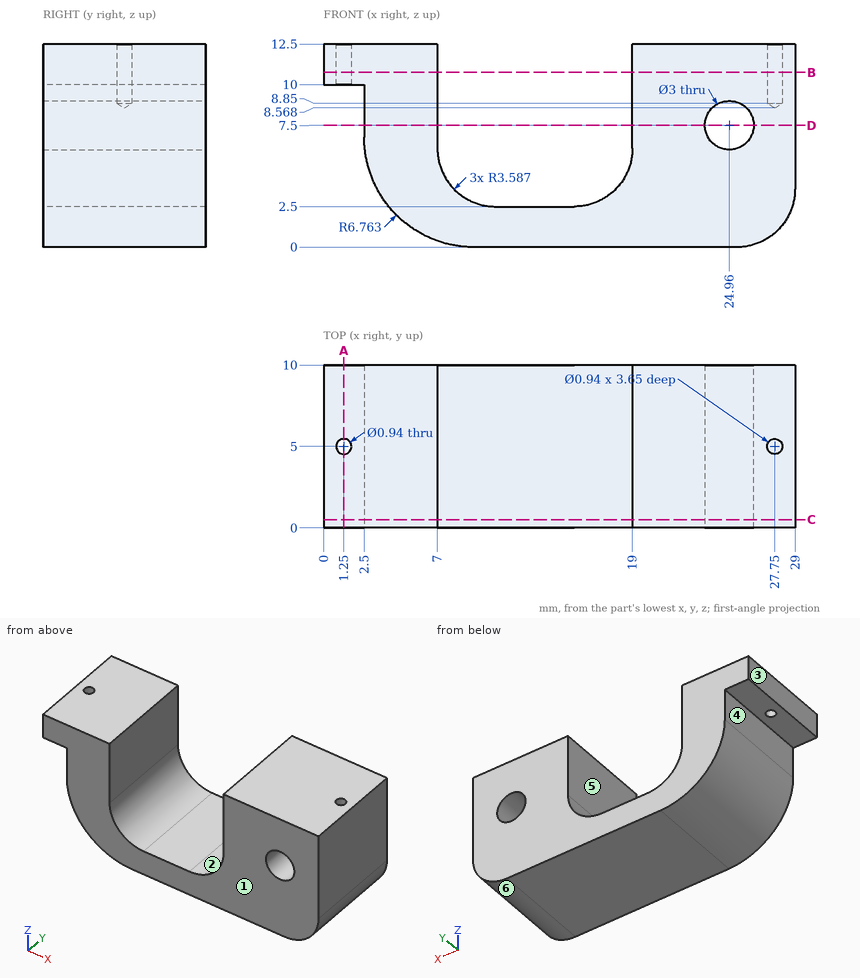
Study the drawing (mm; zero at the part's minimum x, y, z) and answer. A direction names the side the tool comes from. Round coordinates to 2 decimals unless told otherwise and drop trailing zeros. Write each loop counter-clockwise with the first axis right and the second up, starting at its lowest first coordinate (ties: lowest second). Pieces come first, ordered by that corner, then holes. Notation, with made-up numbers: (43, 73.5) - (48, 73.5) arc R19 ccw to (48, 94.5) - close; hole circle Ø4 at (-10.75, 26.25). An arc over 180 degrees is marked (long way). Use a Markdown table: item, result. Add a question column.
1. The part is cut by section C-C (y = 0.5). Write down the section's boundary in (x, z) (1 decimal), and give its area (3 significant figures).
2. The part is cut by section B-B (z = 10.75). Write down the section's boundary in (x, y).
3. The part is cut by section D-D (z = 7.5). Write down the section's boundary in (x, y), and give its area (3 significant figures).
4. The part is cut by section A-A (x = 1.25). Write down the section's boundary in (y, z).
5. Flat-ended cylindrical pins translate along their axes: P1, Ø5.5, axis at x = 13, y = 3, coming from the +Z side; P2, Ø2, axis at x = 8.5, y = 8.5, coming from the +Z side; P3, Ø6, axis at x = 3.5, y = 7.5, coming from the -Z side. Find the tip coordinate at first contact, or state that the pin passes through.
6. A tool of negligible diameter and unlimited length cuts with its end or side. For the marked faces 4, 5 and 6, from which of +Z, -Z, +X, -X, +Y, -Y can it reach the whole face along a straight path? Write none if from no direction.
7. Consider line 1 (X direction, y = 5, z = 10.5); line 2 (Z direction, x = 24.96, y = 3.25); line 3 (Y direction, x = 1.25, z = 11.3). Determine where each line is inside the solid, lowest interval first.
8. For a pull along X with two mould halves and no side action, classify the marked faces 1, 2 and 3 as +X half, -X half, draft (parallel to the pull), parting line (faces both ways), or undercut.
Reported:
| question | item | result |
|---|---|---|
| 1 | outline | (0, 10) - (2.5, 10) - (2.5, 6.8) arc R6.8 ccw to (9.3, 0) - (25.4, 0) arc R3.6 ccw to (29, 3.6) - (29, 12.5) - (19, 12.5) - (19, 6.1) arc R3.6 cw to (15.4, 2.5) - (10.6, 2.5) arc R3.6 cw to (7, 6.1) - (7, 12.5) - (0, 12.5) - close; hole circle Ø3 at (25, 7.5) |
| 1 | area | 203 mm^2 |
| 2 | outline | (0, 0) - (7, 0) - (7, 10) - (0, 10) - close; (19, 0) - (29, 0) - (29, 10) - (19, 10) - close; hole circle Ø0.94 at (1.25, 5); hole circle Ø0.94 at (27.75, 5) |
| 3 | outline | (2.5, 0) - (7, 0) - (7, 10) - (2.5, 10) - close; (19, 0) - (23.46, 0) - (23.46, 10) - (19, 10) - close; (26.46, 0) - (29, 0) - (29, 10) - (26.46, 10) - close |
| 3 | area | 115 mm^2 |
| 4 | outline | (0, 10) - (4.53, 10) - (4.53, 12.5) - (0, 12.5) - close; (5.47, 10) - (10, 10) - (10, 12.5) - (5.47, 12.5) - close |
| 5 | P1 | z = 2.52 |
| 5 | P2 | z = 4.26 |
| 5 | P3 | z = 0.59 |
| 6 | face 4 | -Z, -X, +Y, -Y |
| 6 | face 5 | +Z, +Y, -Y |
| 6 | face 6 | -Z, +X, +Y, -Y |
| 7 | line 1 | 0 to 0.78, 1.72 to 7, 19 to 27.28, 28.22 to 29 |
| 7 | line 2 | 0 to 6, 9 to 12.5 |
| 7 | line 3 | 0 to 4.53, 5.47 to 10 |
| 8 | face 1 | draft |
| 8 | face 2 | undercut |
| 8 | face 3 | -X half |
